Input: part model. Units: mm. Frame: model coordinates. Round coordinates to 2 decimals unless told otherwise and drop trailing zeros. Order: outer loops, then holes, each group sorted by start corner. A loop starts at its lowest first (then second) coordinate and runs counter-clockwise, first axis right, second up. Notation, with made-up numbers: M 28,76.5 L 52,76.5 A10 cw 52,81.5 Z; hole C 54,-37 d10. An arc over 180 degrees is marked long. One line per question, with ' | ' between items.
```python
from build123d import *

# Parameters (mm, degrees)
F0_R     = 34.0839137212
F1_DEPTH = 25.4


with BuildPart() as f1:
    # F0 (on Front) → F1 (new body)
    with BuildSketch(Plane.XZ):
        with BuildLine():
            ThreePointArc((19.3380191922, -53.4293892983), (46.5159637147, -32.6331694256), (56.8212867424, 0))
            ThreePointArc((56.8212867424, 0), (-31.4202012773, 47.3437385381), (-22.0727231354, -52.3588915129))
            Line((-22.0727231354, -52.3588915129), (-22.0727231354, -44.1123396158))
            Line((-22.0727231354, -44.1123396158), (19.3380191922, -44.1123396158))
            Line((19.3380191922, -44.1123396158), (19.3380191922, -53.4293892983))
        make_face()
        Circle(F0_R, mode=Mode.SUBTRACT)
        with BuildLine():
            Line((-22.0727231354, -44.1123396158), (-22.0727231354, -52.3588915129))
            ThreePointArc((-22.0727231354, -52.3588915129), (-1.4683810103, -56.802310554), (19.3380191922, -53.4293892983))
            Line((19.3380191922, -53.4293892983), (19.3380191922, -44.1123396158))
            Line((19.3380191922, -44.1123396158), (-22.0727231354, -44.1123396158))
        make_face()
        with BuildLine():
            ThreePointArc((19.3380191922, -53.4293892983), (-1.4683810103, -56.802310554), (-22.0727231354, -52.3588915129))
            Line((-22.0727231354, -52.3588915129), (-22.0727231354, -107.8437715769))
            Line((-22.0727231354, -107.8437715769), (19.3380191922, -107.8437715769))
            Line((19.3380191922, -107.8437715769), (19.3380191922, -53.4293892983))
        make_face()
    extrude(amount=F1_DEPTH)


solid = f1.part
```
Item 1: Line query: line 1 along Z through (x, y) = (0, -9); line 2 along X through (y, z) = (-7, -94); line 3 along Z through (x, y) = (-2.5, -14.25). Output: solid intervals per line, ascending. Write a range as from..to.
Report:
line 1: -107.84..-34.08, 34.08..56.82 | line 2: -22.07..19.34 | line 3: -107.84..-33.99, 33.99..56.77
Item 2: Section query D-D, the plane z = -61.5. Return loops of the section in (x, y), plus the area to 3 significant figures.
Report:
outline: M -22.07,-25.4 L 19.34,-25.4 L 19.34,0 L -22.07,0 Z | area: 1,050 mm²
Item 3: First-contact query: pin 1 (4 mm diameter, centred on y = -7, z = -63.5, fed in from +X); pin 2 (6 mm diameter, centred on x = 42.5, y = -3, fed in from -Z); pin 3 (4 mm diameter, centred on y = -17.5, z = -12.5, fed in from +X). Flat tips, straight axial feed; report the tip coordinate or a pass-through.
Report:
pin 1: x = 19.34 | pin 2: z = -40.85 | pin 3: x = 55.84
Item 4: Section query A-A, the plane x = 0. Return loops of the section in (y, z), plus the area to 3 significant figures.
Report:
outline: M -25.4,-107.84 L 0,-107.84 L 0,-34.08 L -25.4,-34.08 Z; M -25.4,34.08 L 0,34.08 L 0,56.82 L -25.4,56.82 Z | area: 2,450 mm²
Item 5: Section query C-C, the plane z = -12. Return loops of the section in (x, y), plus the area to 3 significant figures.
Report:
outline: M -55.54,-25.4 L -31.9,-25.4 L -31.9,0 L -55.54,0 Z; M 31.9,-25.4 L 55.54,-25.4 L 55.54,0 L 31.9,0 Z | area: 1,200 mm²
Item 6: Section query B-B, the plane y = -13.5. Return loops of the section in (x, z).
Report:
outline: M -22.07,-107.84 L 19.34,-107.84 L 19.34,-53.43 A56.82 ccw long -22.07,-52.36 Z; hole C 0,0 d68.17
Item 7: Mould query, pull axis X, two halves, no side actions, for faces 1 (the flat face through (19.338, -13, -81)), 2 (the flat face through (-1, 0, -43)), 3 (the cylindrical face through (32.51, -12.52, 10.24)), 4 (the flat face through (-22.073, -13, -80)). Classes: +X half, -X half, draft (parallel to the pull), parting line (faces both ways), or undercut.
Report:
face 1: +X half | face 2: draft | face 3: undercut | face 4: -X half
